Check sheet for the modelled part. Datum: model origin and axes. Units: mm. Face numbers are marked on the shaded views. Coordinates: 2 decimals unless noted, no trailing zeros. Write each loop counter-clockwise with the first axis right and the second up, starting at its lowest first coordinate (ties: lowest second). Pieces come first, ordered by that corner, then holes. Notation, with made-up numbers: (1.25, -11.5) - (7.25, -11.5) arc R24 ccw to (7.25, 6.5) - close; hole circle Ø2 at (-14, 7.5). An arc over 180 degrees is marked (long way). Write each question's results on one line, items separated by ' | '.
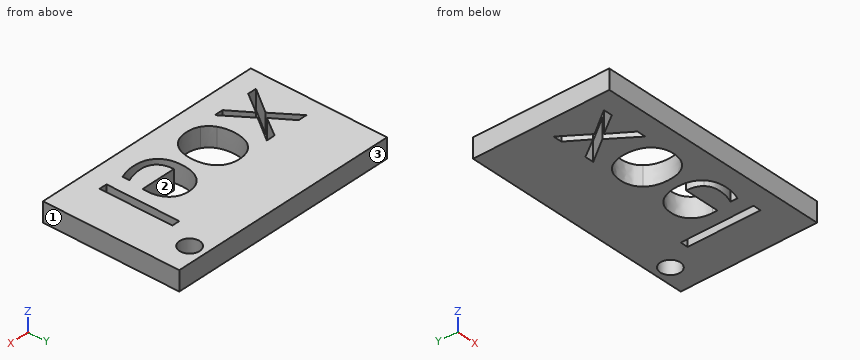
from build123d import *

# Parameters (mm, degrees)
F0_W     = 60
F0_H     = 35
F0_W_2   = 1.9945063705
F0_H_2   = 18.6884094019
F0_R     = 2.5757746771
F1_DEPTH = 5


with BuildPart() as f1:
    # F0 (on Top) → F1 (new body)
    with BuildSketch(Plane.XY):
        with Locations((-30, 17.5)):
            Rectangle(F0_W, F0_H)
        Polygon((-55.554255027, 5.3125368431), (-50.7390016895, 12.0492799403), (-55.3159902969, 18.4747416964), (-53.044789401, 18.4747416964), (-49.5745788952, 13.4327525672), (-46.1158973279, 18.4747416964), (-43.8677543092, 18.4747416964), (-48.4447429165, 12.0492799403), (-43.629489579, 5.3125368431), (-45.8853185567, 5.3125368431), (-49.5745788952, 10.6465924158), (-53.2984260493, 5.3125368431), align=None, mode=Mode.SUBTRACT)
        with BuildLine():
            add(Edge.make_bspline(
                [(-31.2916038326, 16.8779837062), (-29.6641020062, 15.0391180062), (-29.6641020062, 11.9070896981)],
                knots=[0, 0, 0, 1, 1, 1], degree=2))
            add(Edge.make_bspline(
                [(-29.6641020062, 11.9070896981), (-29.6641020062, 8.686672861), (-31.2839178735, 6.8785509972)],
                knots=[0, 0, 0, 1, 1, 1], degree=2))
            add(Edge.make_bspline(
                [(-31.2839178735, 6.8785509972), (-32.9037337409, 5.0704291334), (-35.7629105032, 5.0704291334)],
                knots=[0, 0, 0, 1, 1, 1], degree=2))
            add(Edge.make_bspline(
                [(-35.7629105032, 5.0704291334), (-37.530681082, 5.0704291334), (-38.8987817908, 5.9005127096)],
                knots=[0, 0, 0, 1, 1, 1], degree=2))
            add(Edge.make_bspline(
                [(-38.8987817908, 5.9005127096), (-40.2668824997, 6.7305962857), (-41.0124205264, 8.2793170319)],
                knots=[0, 0, 0, 1, 1, 1], degree=2))
            add(Edge.make_bspline(
                [(-41.0124205264, 8.2793170319), (-41.7579585531, 9.8280377782), (-41.7579585531, 11.9070896981)],
                knots=[0, 0, 0, 1, 1, 1], degree=2))
            add(Edge.make_bspline(
                [(-41.7579585531, 11.9070896981), (-41.7579585531, 15.1236635556), (-40.1477501346, 16.9202564809)],
                knots=[0, 0, 0, 1, 1, 1], degree=2))
            add(Edge.make_bspline(
                [(-40.1477501346, 16.9202564809), (-38.537541716, 18.7168494061), (-35.6783649537, 18.7168494061)],
                knots=[0, 0, 0, 1, 1, 1], degree=2))
            add(Edge.make_bspline(
                [(-35.6783649537, 18.7168494061), (-32.9191056589, 18.7168494061), (-31.2916038326, 16.8779837062)],
                knots=[0, 0, 0, 1, 1, 1], degree=2))
        make_face(mode=Mode.SUBTRACT)
        with BuildLine():
            add(Edge.make_bspline(
                [(-18.3311554041, 5.2702640684), (-19.2726853863, 5.0704291334), (-20.6061992794, 5.0704291334)],
                knots=[0, 0, 0, 1, 1, 1], degree=2))
            add(Edge.make_bspline(
                [(-20.6061992794, 5.0704291334), (-23.5230207345, 5.0704291334), (-25.2120102332, 6.8497286508)],
                knots=[0, 0, 0, 1, 1, 1], degree=2))
            add(Edge.make_bspline(
                [(-25.2120102332, 6.8497286508), (-26.9009997319, 8.6290281682), (-26.9009997319, 11.7841143535)],
                knots=[0, 0, 0, 1, 1, 1], degree=2))
            add(Edge.make_bspline(
                [(-26.9009997319, 11.7841143535), (-26.9009997319, 14.9699443749), (-25.333064088, 16.8433968905)],
                knots=[0, 0, 0, 1, 1, 1], degree=2))
            add(Edge.make_bspline(
                [(-25.333064088, 16.8433968905), (-23.7651284442, 18.7168494061), (-21.121158535, 18.7168494061)],
                knots=[0, 0, 0, 1, 1, 1], degree=2))
            add(Edge.make_bspline(
                [(-21.121158535, 18.7168494061), (-18.6501227042, 18.7168494061), (-17.2090053845, 17.0893475797)],
                knots=[0, 0, 0, 1, 1, 1], degree=2))
            add(Edge.make_bspline(
                [(-17.2090053845, 17.0893475797), (-15.7678880648, 15.4618457533), (-15.7678880648, 12.794817967)],
                knots=[0, 0, 0, 1, 1, 1], degree=2))
            Line((-15.7678880648, 12.794817967), (-15.7678880648, 11.5343206847))
            Line((-15.7678880648, 11.5343206847), (-24.8334767505, 11.5343206847))
            add(Edge.make_bspline(
                [(-24.8334767505, 11.5343206847), (-24.7719890782, 9.2170040346), (-23.6613679972, 8.0160729349)],
                knots=[0, 0, 0, 1, 1, 1], degree=2))
            add(Edge.make_bspline(
                [(-23.6613679972, 8.0160729349), (-22.5507469161, 6.8151418351), (-20.5331826686, 6.8151418351)],
                knots=[0, 0, 0, 1, 1, 1], degree=2))
            add(Edge.make_bspline(
                [(-20.5331826686, 6.8151418351), (-18.4080149944, 6.8151418351), (-16.3328060541, 7.7028701041)],
                knots=[0, 0, 0, 1, 1, 1], degree=2))
            Line((-16.3328060541, 7.7028701041), (-16.3328060541, 5.9235705867))
            add(Edge.make_bspline(
                [(-16.3328060541, 5.9235705867), (-17.3896254219, 5.4700990034), (-18.3311554041, 5.2702640684)],
                knots=[0, 0, 0, 1, 1, 1], degree=2))
        make_face(mode=Mode.SUBTRACT)
        with Locations((-11.369598005, 14.6567415441)):
            Rectangle(F0_W_2, F0_H_2, mode=Mode.SUBTRACT)
        with Locations((-7.4053523131, 31.0702826828)):
            Circle(F0_R, mode=Mode.SUBTRACT)
    extrude(amount=F1_DEPTH)


solid = f1.part
1. Draft check along Y on the marked faces 1, 2 and 3. Enter one of: pulls with the +Y half, pulls with the -Y half, needs draft (parallel to the pull), parting line crosses it, or undercut.
Values follow:
face 1: needs draft | face 2: undercut | face 3: pulls with the +Y half
2. Material ranges on L1, parallel to X at y = 19, z = 1.65; L2, parallel to X at y = 15, z = 0.5; L3, parallel to X at y = 11, z = 2.8, recorded low to high. Write a range as [from, to].
Values follow:
L1: x = [-60, -12.37], [-10.37, 0] | L2: x = [-60, -52.84], [-50.65, -48.5], [-46.34, -41.28], [-30.17, -26.39], [-16.06, -12.37], [-10.37, 0] | L3: x = [-60, -51.49], [-47.69, -41.72], [-29.7, -26.87], [-24.8, -12.37], [-10.37, 0]
3. Go/stop test with a flat-tipped pin: pin 1 (1.8 mm diameter, centred on x = -44.5, z = 2, fed in from -Y). Record where the tip stops, or that it passes through.
Values follow:
pin 1: stops at y = 0
4. Sectioned sample at B-B (x = -22). Give the number of separate pieces and of enclosed holes in the cut face, then the cut area to 3 significant figures.
Values follow:
separate pieces: 3 | enclosed holes: 0 | area: 130 mm^2
5. Sectioned sample at A-A (y = 21.5). Record the cut outline in (x, z).
Values follow:
outline: (-60, 0) - (-12.37, 0) - (-12.37, 5) - (-60, 5) - close; (-10.37, 0) - (0, 0) - (0, 5) - (-10.37, 5) - close
